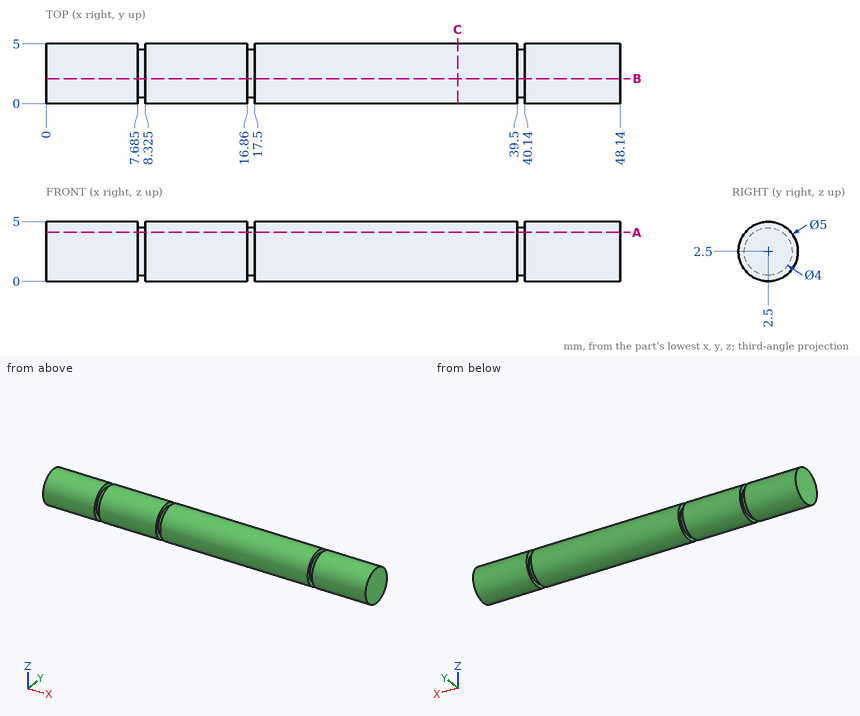
Geometry check sheet. Reference: drawing and pictorial views, mm from the part's lowest x, y, z. Coordinates: 2 decimals unless noted, no trailing zeros. Order: outer loops, then holes, each group sorted by start corner. A loop starts at its lowest first (then second) coordinate and runs counter-clockwise, first axis right, second up.
Item 1: Section check C-C (x = 34.5). Enter the section's corners in (y, z).
Item 2: Section check B-B (y = 2.1). Enter the section's corners in (x, z) (3 decimals), plus the area to 3 significant figures.
Item 3: Section check A-A (z = 4.1). Enter the section's corners in (x, y) (3 decimals), plus the area to 3 significant figures.
Item 4: Scan lines: line 1 along X through (y, z) = (1.55, 4.55) (3 decimals); line 2 along Z through (x, y) = (39, 2.7); line 3 along Z through (x, y) = (24, 1). Record each from-to range of solid material in increasing order.
Check sheet entries:
1. outline: circle Ø5 at (2.5, 2.5)
2. outline: (0, 0.032) - (7.685, 0.032) - (7.685, 0.54) - (8.325, 0.54) - (8.325, 0.032) - (16.86, 0.032) - (16.86, 0.54) - (17.5, 0.54) - (17.5, 0.032) - (39.5, 0.032) - (39.5, 0.54) - (40.14, 0.54) - (40.14, 0.032) - (48.14, 0.032) - (48.14, 4.968) - (40.14, 4.968) - (40.14, 4.46) - (39.5, 4.46) - (39.5, 4.968) - (17.5, 4.968) - (17.5, 4.46) - (16.86, 4.46) - (16.86, 4.968) - (8.325, 4.968) - (8.325, 4.46) - (7.685, 4.46) - (7.685, 4.968) - (0, 4.968) - close
2. area: 236 mm2
3. outline: (0, 0.579) - (7.685, 0.579) - (7.685, 1.3) - (8.325, 1.3) - (8.325, 0.579) - (16.86, 0.579) - (16.86, 1.3) - (17.5, 1.3) - (17.5, 0.579) - (39.5, 0.579) - (39.5, 1.3) - (40.14, 1.3) - (40.14, 0.579) - (48.14, 0.579) - (48.14, 4.421) - (40.14, 4.421) - (40.14, 3.7) - (39.5, 3.7) - (39.5, 4.421) - (17.5, 4.421) - (17.5, 3.7) - (16.86, 3.7) - (16.86, 4.421) - (8.325, 4.421) - (8.325, 3.7) - (7.685, 3.7) - (7.685, 4.421) - (0, 4.421) - close
3. area: 182 mm2
4. line 1: x = 0 to 7.685, 8.325 to 16.86, 17.5 to 39.5, 40.14 to 48.14
4. line 2: z = 0.01 to 4.99
4. line 3: z = 0.5 to 4.5
